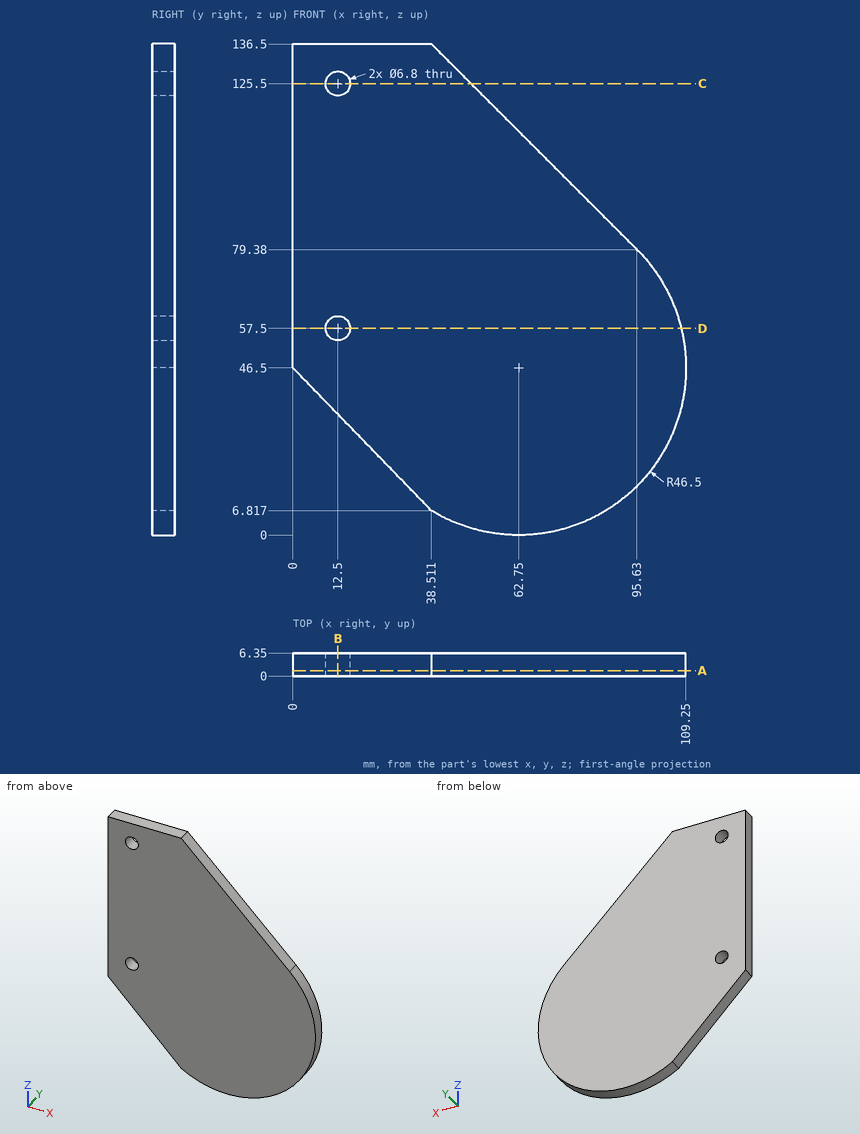
Verification items for this drawing (mm, ordinates from the low corner). Round coordinates to 2 decimals unless told otherwise and drop trailing zeros. Order: outer loops, then holes, each group sorted by start corner. A loop starts at its lowest first (then second) coordinate and runs counter-clockwise, first axis right, second up. Notation, with made-up numbers: (74.5, -39) - (104.5, -39) arc R30 ccw to (104.5, -14) - close; hole circle Ø3 at (69, -5). An arc over 180 degrees is marked (long way). Use CSV: the item, a comma, the result in double quotes. Start each with the question number.
1) Section check A-A, the plane y = 1.5. Record the cut outline in (x, z), plus the area to 3 significant figures.
2) Section check D-D, the plane z = 57.5. Record the cut outline in (x, y).
3) Go/stop test with a flat-tipped pin: P1, Ø1.5, axis at x = 13.5, y = 2.5, coming from the -Z side (1 decimal). Record where the tip stops, or that it passes through.
4) Thickness scan on L1, parallel to Z at x = 38.5, y = 5; L2, parallel to X at y = 3.75, z = 57.5; L3, parallel to X at y = 4, z = 125.5. Record the ranges inside material, lowest first.
5) Section check B-B, the plane x = 12.5. Record the cut outline in (y, z).
6) Section check C-C, the plane z = 125.5. Record the cut outline in (x, y), plus the area to 3 significant figures.
Answers:
1,outline,"(0, 46.5) - (38.51, 6.82) arc R46.5 ccw to (95.63, 79.38) - (38.51, 136.5) - (0, 136.5) - close; hole circle Ø6.8 at (12.5, 57.5); hole circle Ø6.8 at (12.5, 125.5)"
1,area,"10,700 mm²"
2,outline,"(0, 0) - (9.1, 0) - (9.1, 6.35) - (0, 6.35) - close; (15.9, 0) - (107.93, 0) - (107.93, 6.35) - (15.9, 6.35) - close"
3,P1,"stops at z = 31.8"
4,L1,"z = 6.83 to 136.5"
4,L2,"x = 0 to 9.1, 15.9 to 107.93"
4,L3,"x = 0 to 9.1, 15.9 to 49.51"
5,outline,"(0, 33.62) - (6.35, 33.62) - (6.35, 54.1) - (0, 54.1) - close; (0, 60.9) - (6.35, 60.9) - (6.35, 122.1) - (0, 122.1) - close; (0, 128.9) - (6.35, 128.9) - (6.35, 136.5) - (0, 136.5) - close"
6,outline,"(0, 0) - (9.1, 0) - (9.1, 6.35) - (0, 6.35) - close; (15.9, 0) - (49.51, 0) - (49.51, 6.35) - (15.9, 6.35) - close"
6,area,"271 mm²"
